Design review of the part built by this model. Coordinates are the model's own, in mm. Face numbers are marked on the shaded views. Round coordinates to 2 decimals unless told otherwise and drop trailing zeros. Return JSON: item names as keys, results as strings. Group by question number.
(1) Wall thickness on L1, parallel to Z at x = 143, y = 55.5; L2, parallel to Y at x = 74.5, z = 2.25; L3, parallel to Y at x = 65, z = 7.5: over which ranges is each line inside the solid? List them lowest first. Write a range as [from, to].
(2) Clearance check with flat-ended pins moving along their axes: pin 1 (3 mm diameter, centred on x = 73.5, y = 41.01, fed in from +Z); pin 2 (1.8 mm diameter, centred on x = 72, y = 40.5, fed in from +Z); pin 3 (2 mm diameter, centred on x = 102.5, z = 5.5, fed in from -Y). State where each tip first meets the part, or that it passes through.
(3) The part is to be moulded in two halves that separate along Y. For the marked faces 1 and 2, say which applies: pulls with the +Y half, pulls with the -Y half, needs draft (parallel to the pull), parting line crosses it, or undercut.
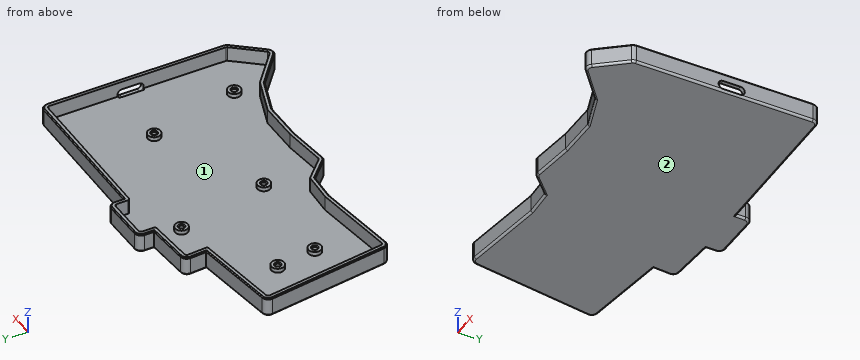
from build123d import *

# Parameters (mm, degrees)
BOSS_EXTRUDE1_DEPTH = 2
BOSS_EXTRUDE2_DEPTH = 9
SKETCH7_R           = 3
SKETCH7_R_2         = 1.100094
SKETCH7_R_3         = 1.100095
SKETCH7_R_4         = 1.14540164
SKETCH7_R_5         = 1.100094267
BOSS_EXTRUDE3_DEPTH = 4
CUT_EXTRUDE1_DEPTH  = 3
FILLET2_R           = 1
CHAMFER1_SIZE       = 0.5
CHAMFER2_SIZE       = 0.5


with BuildPart() as part:
    # Sketch3 → Boss-Extrude1 (new body)
    with BuildSketch(Plane.XY):
        with BuildLine():
            Line((60.855233133, 23.823211938), (47.949977192, 24.377676222))
            Line((47.949977192, 24.377676222), (9.438001399, 18.932389733))
            ThreePointArc((9.438001399, 18.932389733), (7.157815869, 19.520564151), (5.962231275, 21.549300871))
            Line((5.962231275, 21.549300871), (-1.970708405, 77.995680607))
            ThreePointArc((-1.970708405, 77.995680607), (-1.383464331, 80.271537635), (0.639738461, 81.467794829))
            Line((0.639738461, 81.467794829), (38.699898469, 86.902208152))
            Line((38.699898469, 86.902208152), (38.171393284, 94.460167157))
            ThreePointArc((38.171393284, 94.460167157), (38.910984807, 96.683773594), (41.002517903, 97.740613468))
            Line((41.002517903, 97.740613468), (60.921819416, 99.276682226))
            Line((60.921819416, 99.276682226), (60.921819416, 103.721902307))
            ThreePointArc((60.921819416, 103.721902307), (61.804499235, 105.878127499), (63.945786912, 106.796450874))
            Line((63.945786912, 106.796450874), (83.059551455, 107.113531682))
            ThreePointArc((83.059551455, 107.113531682), (85.251859467, 106.245869167), (86.185286941, 104.080744272))
            Line((86.185286941, 104.080744272), (86.24375422, 99.780452187))
            Line((86.24375422, 99.780452187), (154.596820419, 99.780452187))
            ThreePointArc((154.596820419, 99.780452187), (156.771169517, 98.879807301), (157.671814403, 96.705458202))
            Line((157.671814403, 96.705458202), (157.671814403, 14.057773112))
            ThreePointArc((157.671814403, 14.057773112), (157.497078938, 13.035997261), (156.992732263, 12.130352296))
            Line((156.992732263, 12.130352296), (146.547659954, -0.852593653))
            ThreePointArc((146.547659954, -0.852593653), (144.453525054, -1.98521487), (142.178510717, -1.283401812))
            Line((142.178510717, -1.283401812), (127.110775499, 11.324099062))
            Line((127.110775499, 11.324099062), (110.204782414, 17.079131321))
            Line((110.204782414, 17.079131321), (91.635796855, 16.870620568))
            Line((91.635796855, 16.870620568), (72.085555936, 14.46343429))
            ThreePointArc((72.085555936, 14.46343429), (70.725838171, 14.602041008), (69.560483965, 15.316179508))
            Line((69.560483965, 15.316179508), (60.855233133, 23.823211938))
        make_face()
    extrude(amount=BOSS_EXTRUDE1_DEPTH)

    # Sketch4 → Boss-Extrude2 (add)
    with BuildSketch(Plane.XY):
        with BuildLine():
            Line((47.949977192, 24.377676222), (60.855233133, 23.823211938))
            Line((60.855233133, 23.823211938), (69.560483965, 15.316179508))
            ThreePointArc((69.560483965, 15.316179508), (70.725838171, 14.602041008), (72.085555936, 14.46343429))
            Line((72.085555936, 14.46343429), (91.635796855, 16.870620568))
            Line((91.635796855, 16.870620568), (110.204782414, 17.079131321))
            Line((110.204782414, 17.079131321), (127.110775499, 11.324099062))
            Line((127.110775499, 11.324099062), (142.178510717, -1.283401812))
            ThreePointArc((142.178510717, -1.283401812), (144.453525054, -1.98521487), (146.547659954, -0.852593653))
            Line((146.547659954, -0.852593653), (156.992732263, 12.130352296))
            ThreePointArc((156.992732263, 12.130352296), (157.497078938, 13.035997261), (157.671814403, 14.057773112))
            Line((157.671814403, 14.057773112), (157.671814403, 96.705458202))
            ThreePointArc((157.671814403, 96.705458202), (156.771169517, 98.879807301), (154.596820419, 99.780452187))
            Line((154.596820419, 99.780452187), (86.24375422, 99.780452187))
            Line((86.24375422, 99.780452187), (86.185286941, 104.080744272))
            ThreePointArc((86.185286941, 104.080744272), (85.251859467, 106.245869167), (83.059551455, 107.113531682))
            Line((83.059551455, 107.113531682), (63.945786912, 106.796450874))
            ThreePointArc((63.945786912, 106.796450874), (61.804499235, 105.878127499), (60.921819416, 103.721902307))
            Line((60.921819416, 103.721902307), (60.921819416, 99.276682226))
            Line((60.921819416, 99.276682226), (41.002517903, 97.740613468))
            ThreePointArc((41.002517903, 97.740613468), (38.910984807, 96.683773594), (38.171393284, 94.460167157))
            Line((38.171393284, 94.460167157), (38.699898469, 86.902208152))
            Line((38.699898469, 86.902208152), (0.639738461, 81.467794829))
            ThreePointArc((0.639738461, 81.467794829), (-1.383464331, 80.271537635), (-1.970708405, 77.995680607))
            Line((-1.970708405, 77.995680607), (5.962231275, 21.549300871))
            ThreePointArc((5.962231275, 21.549300871), (7.157815869, 19.520564151), (9.438001399, 18.932389733))
            Line((9.438001399, 18.932389733), (47.949977192, 24.377676222))
        make_face()
        with BuildLine():
            ThreePointArc((84.258355662, 98.692914663), (84.533669024, 98.04695842), (85.183308419, 97.780452187))
            Line((85.183308419, 97.780452187), (154.596820419, 97.780452187))
            ThreePointArc((154.596820419, 97.780452187), (155.356955955, 97.465593738), (155.671814403, 96.705458202))
            Line((155.671814403, 96.705458202), (155.671814403, 14.057773112))
            ThreePointArc((155.671814403, 14.057773112), (155.610734868, 13.70060696), (155.434438315, 13.38403486))
            Line((155.434438315, 13.38403486), (144.989366006, 0.401088911))
            ThreePointArc((144.989366006, 0.401088911), (144.257272174, 0.005133041), (143.461944249, 0.250481615))
            Line((143.461944249, 0.250481615), (128.108249423, 13.097251096))
            Line((128.108249423, 13.097251096), (110.524936275, 19.082852408))
            Line((110.524936275, 19.082852408), (91.501949272, 18.869243682))
            Line((91.501949272, 18.869243682), (71.841145237, 16.448443965))
            ThreePointArc((71.841145237, 16.448443965), (71.365754809, 16.496904248), (70.958318613, 16.74658445))
            Line((70.958318613, 16.74658445), (61.958856362, 25.54112911))
            ThreePointArc((61.958856362, 25.54112911), (61.679828995, 25.728441638), (61.352295386, 25.803701118))
            Line((61.352295386, 25.803701118), (47.852081394, 26.383727313))
            Line((47.852081394, 26.383727313), (9.158002316, 20.91269287))
            ThreePointArc((9.158002316, 20.91269287), (8.360780393, 21.118336461), (7.942767807, 21.827644264))
            Line((7.942767807, 21.827644264), (0.009828128, 78.274024))
            ThreePointArc((0.009828128, 78.274024), (0.215128769, 79.069664055), (0.922440855, 79.487875801))
            Line((0.922440855, 79.487875801), (39.972806225, 85.063675424))
            ThreePointArc((39.972806225, 85.063675424), (40.561555536, 85.398058084), (40.76480024, 86.043913413))
            Line((40.76480024, 86.043913413), (40.166521363, 94.599680421))
            ThreePointArc((40.166521363, 94.599680421), (40.425084652, 95.377059525), (41.156290542, 95.746533736))
            Line((41.156290542, 95.746533736), (62.067941403, 97.359127107))
            ThreePointArc((62.067941403, 97.359127107), (62.675544492, 97.652931317), (62.921819416, 98.281303094))
            Line((62.921819416, 98.281303094), (62.921819416, 103.721902307))
            ThreePointArc((62.921819416, 103.721902307), (63.230393236, 104.475691655), (63.978960617, 104.796726017))
            Line((63.978960617, 104.796726017), (83.09272516, 105.113806824))
            ThreePointArc((83.09272516, 105.113806824), (83.859148665, 104.810474928), (84.185471769, 104.053554549))
            Line((84.185471769, 104.053554549), (84.258355662, 98.692914663))
        make_face(mode=Mode.SUBTRACT)
    extrude(amount=BOSS_EXTRUDE2_DEPTH)

    # Sketch7 → Boss-Extrude3 (add)
    # profile 1 of 6: a face of its own
    with BuildSketch(Plane.XY):
        with Locations((25.178343626, 43.435558637)):
            Circle(SKETCH7_R)
        with Locations((25.178343626, 43.435558637)):
            Circle(SKETCH7_R_2, mode=Mode.SUBTRACT)
    # profile 2 of 6: a face of its own
    with BuildSketch(Plane.XY):
        with Locations((22.534055897, 62.250653675)):
            Circle(SKETCH7_R)
        with Locations((22.534055897, 62.250653675)):
            Circle(SKETCH7_R_2, mode=Mode.SUBTRACT)
    # profile 3 of 6: a face of its own
    with BuildSketch(Plane.XY):
        with Locations((63.99681822, 84.705447078)):
            Circle(SKETCH7_R)
        with Locations((63.99681822, 84.705447078)):
            Circle(SKETCH7_R_3, mode=Mode.SUBTRACT)
    # profile 4 of 6: a face of its own
    with BuildSketch(Plane.XY):
        with Locations((73.496822591, 41.005447941)):
            Circle(SKETCH7_R)
        with Locations((73.496822591, 41.005447941)):
            Circle(SKETCH7_R_3, mode=Mode.SUBTRACT)
    # profile 5 of 6: a face of its own
    with BuildSketch(Plane.XY):
        with Locations((124.796820928, 64.405450202)):
            Circle(SKETCH7_R)
        with Locations((124.796820928, 64.405450202)):
            Circle(SKETCH7_R_4, mode=Mode.SUBTRACT)
    # profile 6 of 6: a face of its own
    with BuildSketch(Plane.XY):
        with Locations((134.70931431, 21.546419059)):
            Circle(SKETCH7_R)
        with Locations((134.70931431, 21.546419059)):
            Circle(SKETCH7_R_5, mode=Mode.SUBTRACT)
    extrude(amount=BOSS_EXTRUDE3_DEPTH)

    # Sketch8 → Cut-Extrude1 (cut)
    with BuildSketch(Plane(origin=(157.671814403, 0, 0), x_dir=(0, 0, -1), z_dir=(1, 0, 0))):
        with BuildLine():
            Line((-1, 62.669458202), (-1, 54.541458202))
            ThreePointArc((-1, 54.541458202), (-3.061576359, 52.479881843), (-5.123152718, 54.541458202))
            Line((-5.123152718, 54.541458202), (-5.123152718, 62.669458202))
            ThreePointArc((-5.123152718, 62.669458202), (-3.061576359, 64.731034561), (-1, 62.669458202))
        make_face()
    extrude(amount=-CUT_EXTRUDE1_DEPTH, mode=Mode.SUBTRACT)

    # Fillet2
    fillet2_edges = [part.edges().sort_by_distance(p)[0] for p in [
        (65.207858549, 19.569695723, 0),
        (54.402605163, 24.10044408, 0),
        (28.693989296, 21.655032978, 0),
        (7.157815869, 19.520564151, 0),
        (1.995761435, 49.772490739, 0),
        (-1.383464331, 80.271537635, 0),
        (19.669818465, 84.18500149, 0),
        (38.435645877, 90.681187654, 0),
        (38.910984807, 96.683773594, 0),
        (50.962168659, 98.508647847, 0),
        (60.921819416, 101.499292266, 0),
        (61.804499235, 105.878127499, 0),
        (73.502669184, 106.954991278, 0),
        (85.251859467, 106.245869167, 0),
        (86.21452058, 101.930598229, 0),
        (120.420287319, 99.780452187, 0),
        (156.771169517, 98.879807301, 0),
        (157.671814403, 55.381615657, 0),
        (157.497078938, 13.035997261, 0),
        (151.770196108, 5.638879321, 0),
        (144.453525054, -1.98521487, 0),
        (134.644643108, 5.020348625, 0),
        (118.657778957, 14.201615191, 0),
        (100.920289635, 16.974875944, 0),
        (81.860676395, 15.667027429, 0),
        (70.725838171, 14.602041008, 0),
    ]]
    fillet(fillet2_edges, radius=FILLET2_R - 0.0001)  # a hair under: the kernel refuses the full size

    # Chamfer1
    chamfer1_edges = [part.edges().sort_by_distance(p)[0] for p in [
        (70.725838171, 14.602041008, 9),
        (81.860676395, 15.667027429, 9),
        (100.920289635, 16.974875944, 9),
        (118.657778957, 14.201615191, 9),
        (134.644643108, 5.020348625, 9),
        (144.453525054, -1.98521487, 9),
        (151.770196108, 5.638879321, 9),
        (157.497078938, 13.035997261, 9),
        (157.671814403, 55.381615657, 9),
        (156.771169517, 98.879807301, 9),
        (120.420287319, 99.780452187, 9),
        (86.21452058, 101.930598229, 9),
        (85.251859467, 106.245869167, 9),
        (73.502669184, 106.954991278, 9),
        (61.804499235, 105.878127499, 9),
        (60.921819416, 101.499292266, 9),
        (50.962168659, 98.508647847, 9),
        (38.910984807, 96.683773594, 9),
        (38.435645877, 90.681187654, 9),
        (19.669818465, 84.18500149, 9),
        (-1.383464331, 80.271537635, 9),
        (1.995761435, 49.772490739, 9),
        (7.157815869, 19.520564151, 9),
        (28.693989296, 21.655032978, 9),
        (54.402605163, 24.10044408, 9),
        (65.207858549, 19.569695723, 9),
    ]]
    chamfer(chamfer1_edges, length=CHAMFER1_SIZE)

    # Chamfer2
    chamfer2_edges = [part.edges().sort_by_distance(p)[0] for p in [
        (133.609220043, 21.546419059, 4),
        (123.651419288, 64.405450202, 4),
        (72.396727591, 41.005447941, 4),
        (62.89672322, 84.705447078, 4),
        (21.433961897, 62.250653675, 4),
        (24.078249626, 43.435558637, 4),
    ]]
    chamfer(chamfer2_edges, length=CHAMFER2_SIZE)


solid = part.part
Solutions:
{
 "1": {"L1": "[0, 2]", "L2": "[14.76, 16.78], [38.18, 40.55], [41.46, 43.83], [104.97, 106.97]", "L3": "[19.77, 22.57], [104.81, 106.81]"},
 "2": {"pin 1": "z = 3.91", "pin 2": "z = 4", "pin 3": "y = 16.98"},
 "3": {"face 1": "undercut", "face 2": "needs draft"}
}
